Verification items for the finished model (mm, model axes). A direction names the side the tool comes from. Give positions to 0.01 mm unless a question says otherwise; leave off trailing zeros. Write each loop counter-clockwise with the first axis right and the second up, starting at its lowest first coordinate (ties: lowest second). Pieces come first, ordered by that corner, then holes. Notation, with made-up numbers: (52, 68) - (89, 68) arc R32 ccw to (89, 105) - close; hole circle Ø11 at (74, 74). An arc over 180 degrees is marked (long way). Put each result on its own line as item: value.
from build123d import *

# Parameters (mm, degrees)
SZKIC1_W                        = 71.725484412
SZKIC1_H                        = 102.625
SZKIC1_R                        = 2.7
SZKIC1_R_2                      = 1.5
DODANIE_WYCI_GNI_CIE1_DEPTH     = 5
WYTNIJ_WYCI_GNI_CIE1_START      = 5
WYTNIJ_WYCI_GNI_CIE1_DEPTH      = 3
SZKIC2_R                        = 4.5
WYTNIJ_WYCI_GNI_CIE2_DEPTH      = 2
ZAOKR_GLENIE1_R                 = 5
SFAZOWANIE2_SIZE                = 1
SZKIC4_R                        = 1.75
WYTNIJ_WYCI_GNI_CIE3_DEPTH      = 83.181434095
SZKIC5_R                        = 3.5
WYTNIJ_WYCI_GNI_CIE4_DEPTH      = 2
SFAZOWANIE3_SIZE                = 0.6
SZKIC8_R                        = 2.7
SZKIC8_R_2                      = 1.75
SZKIC8_R_3                      = 1.5
DODANIE_WYCI_GNI_CIE2_DEPTH     = 0.2
WYTNIJ_WYCI_GNI_CIE5_DEPTH      = 167.708717442
WYTNIJ_WYCI_GNI_CIE5_DEPTH_BACK = 167.708717442


with BuildPart() as part:
    # Szkic1 → Dodanie-wyciągnięcie1 (new body)
    with BuildSketch(Plane.XY):
        with Locations((-28.085426569, -0.062784138)):
            Rectangle(SZKIC1_W, SZKIC1_H)
        with Locations((-53.948168775, -41.375284138)):
            Circle(SZKIC1_R, mode=Mode.SUBTRACT)
        with Locations((-2.222684363, -41.375284138)):
            Circle(SZKIC1_R, mode=Mode.SUBTRACT)
        with Locations((-2.222684363, 41.249715862)):
            Circle(SZKIC1_R, mode=Mode.SUBTRACT)
        with BuildLine():
            Line((-22.230303443, 29.274715862), (-22.730303443, 29.274715862))
            Line((-22.730303443, 29.274715862), (-22.730303443, 9.024715862))
            Line((-22.730303443, 9.024715862), (-22.230303443, 9.024715862))
            Line((-22.230303443, 9.024715862), (-22.230303443, 7.424715862))
            Line((-22.230303443, 7.424715862), (-22.730303443, 7.424715862))
            Line((-22.730303443, 7.424715862), (-22.730303443, -2.475284138))
            ThreePointArc((-22.730303443, -2.475284138), (-23.433247168, -4.172340413), (-25.130303443, -4.875284138))
            Line((-25.130303443, -4.875284138), (-35.845303443, -4.875284138))
            Line((-35.845303443, -4.875284138), (-35.845303443, -5.375284138))
            Line((-35.845303443, -5.375284138), (-37.445303443, -5.375284138))
            Line((-37.445303443, -5.375284138), (-37.445303443, -4.875284138))
            Line((-37.445303443, -4.875284138), (-48.160303443, -4.875284138))
            ThreePointArc((-48.160303443, -4.875284138), (-49.857359718, -4.172340413), (-50.560303443, -2.475284138))
            Line((-50.560303443, -2.475284138), (-50.560303443, 7.424715862))
            Line((-50.560303443, 7.424715862), (-51.060303443, 7.424715862))
            Line((-51.060303443, 7.424715862), (-51.060303443, 9.024715862))
            Line((-51.060303443, 9.024715862), (-50.560303443, 9.024715862))
            Line((-50.560303443, 9.024715862), (-50.560303443, 29.274715862))
            Line((-50.560303443, 29.274715862), (-51.060303443, 29.274715862))
            Line((-51.060303443, 29.274715862), (-51.060303443, 30.874715862))
            Line((-51.060303443, 30.874715862), (-50.560303443, 30.874715862))
            Line((-50.560303443, 30.874715862), (-50.560303443, 36.946288737))
            ThreePointArc((-50.560303443, 36.946288737), (-50.377614321, 37.864728975), (-49.857359718, 38.643345012))
            Line((-49.857359718, 38.643345012), (-46.028932593, 42.471772136))
            ThreePointArc((-46.028932593, 42.471772136), (-45.250316556, 42.99202674), (-44.331876318, 43.174715862))
            Line((-44.331876318, 43.174715862), (-37.445303443, 43.174715862))
            Line((-37.445303443, 43.174715862), (-37.445303443, 43.674715862))
            Line((-37.445303443, 43.674715862), (-35.845303443, 43.674715862))
            Line((-35.845303443, 43.674715862), (-35.845303443, 43.174715862))
            Line((-35.845303443, 43.174715862), (-28.958730568, 43.174715862))
            ThreePointArc((-28.958730568, 43.174715862), (-28.04029033, 42.99202674), (-27.261674293, 42.471772136))
            Line((-27.261674293, 42.471772136), (-23.433247168, 38.643345012))
            ThreePointArc((-23.433247168, 38.643345012), (-22.912992565, 37.864728975), (-22.730303443, 36.946288737))
            Line((-22.730303443, 36.946288737), (-22.730303443, 30.874715862))
            Line((-22.730303443, 30.874715862), (-22.230303443, 30.874715862))
            Line((-22.230303443, 30.874715862), (-22.230303443, 29.274715862))
        make_face(mode=Mode.SUBTRACT)
        with Locations((-16.645303443, 19.149715862)):
            Circle(SZKIC1_R_2, mode=Mode.SUBTRACT)
        with Locations((-56.645303443, 19.149715862)):
            Circle(SZKIC1_R_2, mode=Mode.SUBTRACT)
    extrude(amount=DODANIE_WYCI_GNI_CIE1_DEPTH)

    # Szkic1<3> → Wytnij-wyciągnięcie1 (cut)
    with BuildSketch(Plane.XY.offset(WYTNIJ_WYCI_GNI_CIE1_START)):
        with BuildLine():
            Line((-51.593316248, 47.101803403), (-61.418230337, 20.001803403))
            ThreePointArc((-61.418230337, 20.001803403), (-61.567922523, 19.149715862), (-61.418230337, 18.297628321))
            Line((-61.418230337, 18.297628321), (-51.593316248, -8.802371679))
            ThreePointArc((-51.593316248, -8.802371679), (-50.678240322, -9.997259816), (-49.243008434, -10.450284138))
            Line((-49.243008434, -10.450284138), (-24.047598452, -10.450284138))
            ThreePointArc((-24.047598452, -10.450284138), (-22.612366563, -9.997259816), (-21.697290637, -8.802371679))
            Line((-21.697290637, -8.802371679), (-11.872376548, 18.297628321))
            ThreePointArc((-11.872376548, 18.297628321), (-11.722684363, 19.149715862), (-11.872376548, 20.001803403))
            Line((-11.872376548, 20.001803403), (-21.697290637, 47.101803403))
            ThreePointArc((-21.697290637, 47.101803403), (-22.612366563, 48.29669154), (-24.047598452, 48.749715862))
            Line((-24.047598452, 48.749715862), (-49.243008434, 48.749715862))
            ThreePointArc((-49.243008434, 48.749715862), (-50.678240322, 48.29669154), (-51.593316248, 47.101803403))
        make_face()
    extrude(amount=-WYTNIJ_WYCI_GNI_CIE1_DEPTH, mode=Mode.SUBTRACT)

    # Szkic2 → Wytnij-wyciągnięcie2 (cut)
    with BuildSketch(Plane.XY.offset(5)):
        with Locations((-2.222684363, 41.249715862)):
            Circle(SZKIC2_R)
        with Locations((-2.222684363, -41.375284138)):
            Circle(SZKIC2_R)
        with Locations((-53.948168775, -41.375284138)):
            Circle(SZKIC2_R)
    extrude(amount=-WYTNIJ_WYCI_GNI_CIE2_DEPTH, mode=Mode.SUBTRACT)

    # Zaokrąglenie1
    zaokr_glenie1_edges = [part.edges().sort_by_distance(p)[0] for p in [
        (-63.948168775, 51.249715862, 2.5),
        (7.777315637, 51.249715862, 2.5),
        (7.777315637, -51.375284138, 2.5),
        (-63.948168775, -51.375284138, 2.5),
    ]]
    fillet(zaokr_glenie1_edges, radius=ZAOKR_GLENIE1_R)

    # Sfazowanie2
    sfazowanie2_edges = [part.edges().sort_by_distance(p)[0] for p in [
        (-6.722684363, 41.249715862, 5),
        (-6.722684363, -41.375284138, 5),
        (-58.448168775, -41.375284138, 5),
    ]]
    chamfer(sfazowanie2_edges, length=SFAZOWANIE2_SIZE)

    # Szkic4 → Wytnij-wyciągnięcie3 (cut, through all)
    with BuildSketch(Plane(origin=(0, 0, 0), x_dir=(-1, 0, 0), z_dir=(0, 0, -1))):
        with Locations((15.472684363, -5.450284138)):
            Circle(SZKIC4_R)
        with Locations(Location((15.472684363, 43.749715862, 0), (0, 0, 180))):
            Circle(SZKIC4_R)
        with Locations((57.817922523, 43.749715862)):
            Circle(SZKIC4_R)
        with Locations((57.817922523, -5.450284138)):
            Circle(SZKIC4_R)
    extrude(amount=-WYTNIJ_WYCI_GNI_CIE3_DEPTH, mode=Mode.SUBTRACT)

    # Szkic5 → Wytnij-wyciągnięcie4 (cut)
    with BuildSketch(Plane.XY.offset(5)):
        with Locations((-15.472684363, 43.749715862)):
            Circle(SZKIC5_R)
        with Locations((-15.472684363, -5.450284138)):
            Circle(SZKIC5_R)
        with Locations((-57.817922523, -5.450284138)):
            Circle(SZKIC5_R)
        with Locations((-57.817922523, 43.749715862)):
            Circle(SZKIC5_R)
    extrude(amount=-WYTNIJ_WYCI_GNI_CIE4_DEPTH, mode=Mode.SUBTRACT)

    # Sfazowanie3
    sfazowanie3_edges = [part.edges().sort_by_distance(p)[0] for p in [
        (-16.784833593, 4.747628321, 5),
        (-36.645303443, -10.450284138, 5),
        (-56.505773293, 4.747628321, 5),
        (-56.505773293, 33.551803403, 5),
        (-36.645303443, 48.749715862, 5),
        (-16.784833593, 33.551803403, 5),
        (-11.722684363, 19.149715862, 5),
        (-22.612366563, 48.29669154, 5),
        (-50.678240322, 48.29669154, 5),
        (-61.567922523, 19.149715862, 5),
        (-50.678240322, -9.997259816, 5),
        (-22.612366563, -9.997259816, 5),
        (-28.085426569, -51.375284138, 5),
        (-63.948168775, -0.062784138, 5),
        (7.777315637, -0.062784138, 5),
        (-28.085426569, 51.249715862, 5),
        (-62.48370268, 49.785249768, 5),
        (6.312849543, 49.785249768, 5),
        (6.312849543, -49.910818044, 5),
        (-62.48370268, -49.910818044, 5),
    ]]
    chamfer(sfazowanie3_edges, length=SFAZOWANIE3_SIZE)

    # Szkic8 → Dodanie-wyciągnięcie2 (add)
    with BuildSketch(Plane(origin=(0, 0, 0), x_dir=(-1, 0, 0), z_dir=(0, 0, -1))):
        with Locations((2.222684363, -41.375284138)):
            Circle(SZKIC8_R)
        with Locations((53.948168775, -41.375284138)):
            Circle(SZKIC8_R)
        with Locations((2.222684363, 41.249715862)):
            Circle(SZKIC8_R)
        with Locations((57.817922523, 43.749715862)):
            Circle(SZKIC8_R_2)
        with Locations((56.645303443, 19.149715862)):
            Circle(SZKIC8_R_3)
        with Locations((57.817922523, -5.450284138)):
            Circle(SZKIC8_R_2)
        with Locations((15.472684363, -5.450284138)):
            Circle(SZKIC8_R_2)
        with Locations((16.645303443, 19.149715862)):
            Circle(SZKIC8_R_3)
        with Locations((15.472684363, 43.749715862)):
            Circle(SZKIC8_R_2)
    extrude(amount=-DODANIE_WYCI_GNI_CIE2_DEPTH)


with BuildPart() as body_2:
    # Lustro1: mirrored copy
    add(part.part.mirror(Plane(origin=(0, 51.249715862, 5), x_dir=(0, 0, 1), z_dir=(0, -1, 0))))


with BuildPart() as part_1:
    add(part.part)

    # Szkic9 → Wytnij-wyciągnięcie5 (cut, two sides: drawn at the far end of the back side and taken through both)
    with BuildSketch(Plane(origin=(0, 0, 0), x_dir=(-1, 0, 0), z_dir=(0, 0, -1)).offset(-WYTNIJ_WYCI_GNI_CIE5_DEPTH_BACK)):
        with BuildLine():
            Line((-2.777315637, -51.375284138), (58.948168775, -51.375284138))
            ThreePointArc((58.948168775, -51.375284138), (62.48370268, -49.910818044), (63.948168775, -46.375284138))
            Line((63.948168775, -46.375284138), (63.948168775, 46.249715862))
            ThreePointArc((63.948168775, 46.249715862), (62.48370268, 49.785249768), (58.948168775, 51.249715862))
            Line((58.948168775, 51.249715862), (-2.777315637, 51.249715862))
            ThreePointArc((-2.777315637, 51.249715862), (-6.312849543, 49.785249768), (-7.777315637, 46.249715862))
            Line((-7.777315637, 46.249715862), (-7.777315637, -46.375284138))
            ThreePointArc((-7.777315637, -46.375284138), (-6.312849543, -49.910818044), (-2.777315637, -51.375284138))
        make_face()
    extrude(amount=WYTNIJ_WYCI_GNI_CIE5_DEPTH + WYTNIJ_WYCI_GNI_CIE5_DEPTH_BACK, mode=Mode.SUBTRACT)


solid = body_2.part
Q1. Section check B-B, the plane y = 99. Record the cut outline in (x, z).
Answers follow:
outline: (-63.95, 0) - (-50.56, 0) - (-50.56, 2) - (-56.05, 2) - (-56.05, 4.4) - (-56.69, 5) - (-63.35, 5) - (-63.95, 4.4) - close; (-22.73, 0) - (7.78, 0) - (7.78, 4.4) - (7.18, 5) - (-16.6, 5) - (-17.24, 4.4) - (-17.24, 2) - (-22.73, 2) - close
Q2. Scan lines: line 1 along Y through (x, z) = (-4.5, 1.15); line 2 along X through (y, z) = (87, 0.75); line 3 along Y through (x, z) = (-36.5, 1.5). Record each from-to range of solid material in increasing order.
Answers follow:
line 1: y = 51.25 to 59.8, 62.7 to 142.42, 145.33 to 153.87
line 2: x = -63.95 to -50.56, -22.73 to 7.78
line 3: y = 51.25 to 58.82, 107.87 to 153.87
Q3. Section check A-A, the plane x = -38.5. Record the cut outline in (y, z).
Answers follow:
outline: (51.25, 0) - (59.32, 0) - (59.32, 2) - (53.75, 2) - (53.75, 4.4) - (53.15, 5) - (51.85, 5) - (51.25, 4.4) - close; (107.37, 0) - (153.87, 0) - (153.87, 4.4) - (153.27, 5) - (113.55, 5) - (112.95, 4.4) - (112.95, 2) - (107.37, 2) - close
Q4. Go/stop test with flat-tipped pins: pin 1 Ø0.9 at (x, y) = (-16, 83.5) entering from +Z; pin 2 Ø6.5 at (x, y) = (-15.47, 58.75) entering from +Z. Record where each tip stops, or that it passes through.
Answers follow:
pin 1: stops at z = 0.2
pin 2: stops at z = 3
Q5. Release check for a two-part mould opening along X. For faces 4 (the face through (-62.216, 152.071, 4.829)), 5 (the face through (-36, 53.75, 3)) record: released by +X, released by -X, zero draft, split by the parting line, or undercut.
Answers follow:
face 4: released by -X
face 5: undercut
Q6. Set-up check for faces 1 (the face through (-62.522, 152.371, 2.231)), 2 (the face through (-50.56, 100, 1)), 3 (the face through (-54.585, 109.29, 4.014)): record each of +Z, -Z, +X, -X, +Y, -Y from which the full face is reachable in a straight line by a thin tool's end or side.
Answers follow:
face 1: +Z, -Z, -X, +Y
face 2: +Z, -Z
face 3: +Z
Q7. Section check C-C, the plane z = 1. Give the number of separate pieces and of enclosed holes in the cut face, plus the area to 3 significant figures.
Answers follow:
separate pieces: 1
enclosed holes: 10
area: 5,910 mm2
